Check sheet for the modelled part. Datum: model origin and axes. Units: mm. A direction names the side the tool comes from. Give positions to 0.01 mm unless a question says otherwise; leave off trailing zeros. Order: outer loops, then holes, each group sorted by start corner. A loop starts at its lowest first (then second) coordinate and runs counter-clockwise, first axis right, second up. Notation, with made-up numbers: M -30,25 L -21,25 A27 cw -21,44 Z; hole C -37.5,-36.5 d5. An arc over 180 degrees is marked long. Return JSON: item names as keys, results as strings. Group by question number.
from build123d import *

# Parameters (mm, degrees)
SKETCH1_W           = 90
SKETCH1_H           = 45
BOSS_EXTRUDE1_DEPTH = 50
SHELL1_T            = -2
SKETCH13_W          = 41.406561997
SKETCH13_H          = 5
BOSS_EXTRUDE3_DEPTH = 10
SKETCH15_W          = 41
SKETCH15_H          = 5
BOSS_EXTRUDE4_DEPTH = 10
SKETCH11_W          = 41
SKETCH11_H          = 15
CUT_EXTRUDE1_DEPTH  = 3
SKETCH26_R          = 2.5
BOSS_EXTRUDE5_DEPTH = 10
BOSS_EXTRUDE5_TAPER = 3
SKETCH27_R          = 2.5
BOSS_EXTRUDE6_DEPTH = 10
BOSS_EXTRUDE6_TAPER = 3


with BuildPart() as part:
    # Sketch1 → Boss-Extrude1 (new body)
    with BuildSketch(Plane(origin=(0, 0, 0), x_dir=(1, 0, 0), z_dir=(0, 1, 0))):
        with Locations((4.862356655, 3.4550978)):
            Rectangle(SKETCH1_W, SKETCH1_H)
    extrude(amount=BOSS_EXTRUDE1_DEPTH)

    # Shell1
    shell1_openings = [part.faces().sort_by_distance(p)[0] for p in [
        (4.862356655, 50, -3.4550978),
    ]]
    offset(amount=SHELL1_T, openings=shell1_openings, kind=Kind.INTERSECTION)

    # Sketch13 → Boss-Extrude3 (add)
    with BuildSketch(Plane(origin=(-38.137643345, 0, 0), x_dir=(0, 0, -1), z_dir=(1, 0, 0))):
        with Locations((3.658378798, 19.5)):
            Rectangle(SKETCH13_W, SKETCH13_H)
    extrude(amount=BOSS_EXTRUDE3_DEPTH)

    # Sketch15 → Boss-Extrude4 (add)
    with BuildSketch(Plane.ZY.offset(-47.862356655)):
        with Locations((-3.4550978, 24.5)):
            Rectangle(SKETCH15_W, SKETCH15_H)
    extrude(amount=BOSS_EXTRUDE4_DEPTH)

    # Sketch11 → Cut-Extrude1 (cut)
    with BuildSketch(Plane(origin=(-38.137643345, 0, 0), x_dir=(0, 0, -1), z_dir=(1, 0, 0))):
        with Locations((3.4550978, 9.5)):
            Rectangle(SKETCH11_W, SKETCH11_H)
    extrude(amount=-CUT_EXTRUDE1_DEPTH, mode=Mode.SUBTRACT)

    # Sketch26 → Boss-Extrude5 (add)
    with BuildSketch(Plane(origin=(0, 27, 0), x_dir=(1, 0, 0), z_dir=(0, 1, 0))):
        with Locations((42.895820428, 16.185162885)):
            Circle(SKETCH26_R)
    extrude(amount=BOSS_EXTRUDE5_DEPTH, taper=BOSS_EXTRUDE5_TAPER)

    # Sketch27 → Boss-Extrude6 (add)
    with BuildSketch(Plane(origin=(0, 27, 0), x_dir=(1, 0, 0), z_dir=(0, 1, 0))):
        with Locations((42.882046205, -9.342272768)):
            Circle(SKETCH27_R)
    extrude(amount=BOSS_EXTRUDE6_DEPTH, taper=BOSS_EXTRUDE6_TAPER)


solid = part.part
1) Release check for a two-part mould opening along Y. For faces 4 (the face through (43, 22, -4)), 5 (the face through (-28.138, 20, -3)), 6 (the face through (43, 27, -4)) record: released by +Y, released by -Y, zero draft, split by the parting line, or undercut.
2) Sectioned sample at B-B on z = 4. Record the boundary of the cut face in (x, y), then the cut area to 3 significant figures.
3) Tool access check on faces 1 (the face through (-34, 17, -3)), 2 (the face through (47.862, 12, -3)), 3 (the face through (47.862, 38, -3)). Record the directions out of +Z, -Z, +X, -X, +Y, -Y that give a thin tool (end or side, any length) a straight path to the whole face; none if there is none.
4) Sectioned sample at D-D on y = 15. Record the boundary of the cut face in (x, z), then the cut area to 3 significant figures.
5) Depth check by flat-ended pin: P1, Ø5, axis at x = 13.5, z = -15, coming from the +Y side; P2, Ø5, axis at x = -34.5, z = -5.5, coming from the +Y side; P3, Ø1.2, axis at x = 43, z = 10, coming from the +Y side. Enter the tip coordinate at first touch or a pass-through.
6) Sectioned sample at C-C on x = -29.5. Record the boundary of the cut face in (y, z), then the cut area to 3 significant figures.
7) Sectioned sample at A-A on y = 47.5. Record the boundary of the cut face in (x, z).
8) Material ranges on line 1 along Y through (x, z) = (-32.5, -15); line 2 along X through (y, z) = (30.5, -23); line 3 along Z through (x, y) = (-2, 9.5), recorded low to high.
Reply:
{
 "1": {"face 4": "undercut", "face 5": "zero draft", "face 6": "released by +Y"},
 "2": {"outline": "M -40.14,0 L 49.86,0 L 49.86,50 L 47.86,50 L 47.86,27 L 37.86,27 L 37.86,22 L 47.86,22 L 47.86,2 L -40.14,2 Z; M -40.14,17 L -28.14,17 L -28.14,22 L -38.14,22 L -38.14,50 L -40.14,50 Z", "area": "442 mm^2"},
 "3": {"face 1": "-X", "face 2": "none", "face 3": "+Y"},
 "4": {"outline": "M -40.14,-25.96 L 49.86,-25.96 L 49.86,19.04 L -40.14,19.04 L -40.14,17.04 L 47.86,17.04 L 47.86,-23.96 L -40.14,-23.96 Z", "area": "442 mm^2"},
 "5": {"P1": "y = 2", "P2": "y = 22", "P3": "y = 37"},
 "6": {"outline": "M 0,-25.96 L 50,-25.96 L 50,-23.96 L 22,-23.96 L 22,17.04 L 50,17.04 L 50,19.04 L 0,19.04 Z; hole M 2,-23.96 L 17,-23.96 L 17,17.04 L 2,17.04 Z", "area": "487 mm^2"},
 "7": {"outline": "M -40.14,-25.96 L 49.86,-25.96 L 49.86,19.04 L -40.14,19.04 Z; hole M -38.14,-23.96 L 47.86,-23.96 L 47.86,17.04 L -38.14,17.04 Z"},
 "8": {"line 1": "0 to 2, 17 to 22", "line 2": "-40.14 to -38.14, 47.86 to 49.86", "line 3": "-25.96 to -23.96, 17.04 to 19.04"}
}
